Part model, mm, in its own coordinate system. A direction names the side the tool comes from. Round coordinates to 2 decimals unless told otherwise and drop trailing zeros. Loops run counter-clockwise (first coordinate to the right, second up) from the corner with the lowest first, then second, coordinate; pieces in that order, holes last.
from build123d import *

# Parameters (mm, degrees)
SKETCH002_R   = 5
SKETCH002_R_2 = 2.25
PAD002_DEPTH  = 2
PAD003_DEPTH  = 4


with BuildPart() as part:
    # Sketch002 → Pad002 (new body)
    with BuildSketch(Plane.XZ):
        Circle(SKETCH002_R)
        Circle(SKETCH002_R_2, mode=Mode.SUBTRACT)
    extrude(amount=PAD002_DEPTH)

    # Sketch003 (on Face4 of Pad002) → Pad003 (join)
    with BuildSketch(Plane.XZ.offset(2)):
        Polygon((2.5, -4.330127), (5, 0), (2.5, 4.330127), (-2.5, 4.330127), (-5, 0), (-2.5, -4.330127), align=None)
        Polygon((-2, -3.464102), (2, -3.464102), (4, 0), (2, 3.464102), (-2, 3.464102), (-4, 0), align=None, mode=Mode.SUBTRACT)
    extrude(amount=PAD003_DEPTH)


with BuildPart() as part_1:
    # Body001 placement: moved
    add(part.part.moved(Location((20, 146, 61))))


solid = part_1.part
1) Tool access for faces 4 (the face through (17.014, 142.028, 62.756)), 5 (the face through (16, 144, 58.7)), 6 (the face through (16.27, 142.03, 63.2)), 7 (the face through (23.77, 142.03, 63.13)), 8 (the face through (24, 144, 58.7)): list every direction of +Z, -Z, +X, -X, +Y, -Y with a clear straight run to the whole face (end or side of a thin tool).
Values:
face 4: -Y
face 5: -Z, -X, -Y
face 6: +Z, -X, -Y
face 7: +Z, +X, -Y
face 8: -Z, +X, -Y
2) Slice it at C-C, the plane z = 63. Give the cut face in (x, y).
Values:
outline: (15.42, 144) - (16.15, 144) - (16.15, 140) - (17.15, 140) - (17.15, 144) - (18.97, 144) - (18.97, 146) - (15.42, 146) - close; (21.03, 144) - (22.85, 144) - (22.85, 140) - (23.85, 140) - (23.85, 144) - (24.58, 144) - (24.58, 146) - (21.03, 146) - close
3) Mould opens along Z. For faces 1 (the face through (16.986, 142.028, 59.292)), 2 (the face through (16.23, 142.03, 58.87)), 3 (the face through (24, 144, 63.3)) say: released by +Z, released by -Z, zero draft, split by the parting line, or undercut.
Values:
face 1: undercut
face 2: released by -Z
face 3: zero draft
4) Slice it at B-B, the plane x = 20. Give the cut face in (y, z).
Values:
outline: (140, 56.67) - (144, 56.67) - (144, 56) - (146, 56) - (146, 58.75) - (144, 58.75) - (144, 57.54) - (140, 57.54) - close; (140, 64.46) - (144, 64.46) - (144, 63.25) - (146, 63.25) - (146, 66) - (144, 66) - (144, 65.33) - (140, 65.33) - close
5) Slice it at A-A, the plane y = 143.7. Give the cut face in (x, z).
Values:
outline: (15, 61) - (17.5, 56.67) - (22.5, 56.67) - (25, 61) - (22.5, 65.33) - (17.5, 65.33) - close; hole (16, 61) - (18, 57.54) - (22, 57.54) - (24, 61) - (22, 64.46) - (18, 64.46) - close
6) Slice it at D-D, the plane z = 58.5. Give the cut face in (x, y).
Values:
outline: (15.67, 144) - (16.44, 144) - (16.44, 140) - (17.44, 140) - (17.44, 144) - (22.56, 144) - (22.56, 140) - (23.56, 140) - (23.56, 144) - (24.33, 144) - (24.33, 146) - (15.67, 146) - close
7) Wall check: line 1 along Z through (x, y) = (20, 145.5); line 2 along Z through (x, y) = (19.75, 140.3); line 3 along Y through (x, z) = (22, 64). Give the ranges that are in metal, low to high.
Values:
line 1: z = 56 to 58.75, 63.25 to 66
line 2: z = 56.67 to 57.54, 64.46 to 65.33
line 3: y = 144 to 146
8) Drop flat-ended pins along their axis: pin 1 Ø1.5 at (x, y) = (17, 141.5) entering from +Z; pin 2 Ø1 at (x, z) = (21, 60.5) entering from +Y; pin 3 Ø1.2 at (x, z) = (15.5, 58.5) entering from -Y; pin 4 Ø1.2 at (x, y) = (19.5, 142.5) entering from -Z. Give the stop position or say it passes through.
Values:
pin 1: stops at z = 65.33
pin 2: passes through
pin 3: stops at y = 144
pin 4: stops at z = 56.67
